Part model, mm, in its own coordinate system. A direction names the side the tool comes from. Round coordinates to 2 decimals unless told otherwise and drop trailing zeros. Loops run counter-clockwise (first coordinate to the right, second up) from the corner with the lowest first, then second, coordinate; pieces in that order, holes last. Notation, with made-up numbers: M 1.5,35 L 57.5,35 A30 ccw 57.5,59 Z; hole C 13.5,4 d3. An arc over 180 degrees is marked long. Answer as CSV lines item,"result". Start each with the question number.
Item 1: Mould opens along X. For faces 1 (the flat face through (0, -30.48, 2)), 2 (the cylindrical face through (-0.34, -33.61, 1.55)), 3 (the flat face through (12, -3.175, 26)) say: pulls with the +X half, pulls with the -X half, needs draft (parallel to the pull), parting line crosses it, or undercut.
Item 2: Band-saw the part on C-C (y = -33). Give the cut face in (x, z) (1 decimal).
Item 3: Band-saw the part on B-B (z = 16.5). Give the cut face in (x, y) (3 decimals).
Item 4: Drop flat-ended pins along their axis: pin 1 Ø5 at (x, y) = (-5.5, -15.5) entering from +Z; pin 2 Ø1 at (y, z) = (-27, 5.5) entering from +X; pin 3 Ø4 at (x, z) = (16.5, 2.5) entering from -Y. Give the stop position or say it passes through.
Item 5: Wall check: line 1 (X direction, y = 1.45, z = 0); line 2 (Y direction, x = -3.5, z = -3). Give the ranges that are in metal, low to high.
Item 6: Which spindle directions (+Z, -Z, +X, -X, +Y, -Y) get a long thin tool onto all of the face, cutting with end or side? Do faces 4 (the flat face through (6, 3.175, 25)), 5 (the flat face through (0, 0, 0)). Say none if no direction does.
Item 7: Band-saw the part on D-D (x = -10). Give the cut face in (y, z) (3 decimals).
Autodesk Inventor part; units mm, degrees
ref_plane "YZ Plane" through (0, 0, 0) normal (1, 0, 0) x (0, 1, 0)
ref_plane "XZ Plane" through (0, 0, 0) normal (0, 1, 0) x (-1, 0, 0)
ref_plane "XY Plane" through (0, 0, 0) normal (0, 0, 1) x (1, 0, 0)
sketch "Sketch1" plane through (0, 0, 0) normal (0, 1, 0) x (-1, 0, 0)
  arc A0 (-31.75, 0) -> (31.75, 0) centre (0, 0) ccw
  line L0 (0, 0) -> (-31.75, 0) construction
  line L1 (0, 0) -> (31.75, 0) construction
  line L2 (31.75, 0) -> (-31.75, 0)
  dimension "d0" = 31.75
  dimension "d1" = 180
revolve "Revolution1" add sketch "Sketch1" angle 180 about axis through (-31.75, 0, 0) along (-1, 0, 0)
sketch "Sketch2" plane through (0, 0, 0) normal (0, 1, 0) x (1, 0, 0)
  line L0 (0, 0) -> (0, 27.94)
  line L1 (0, 27.94) -> (0, 0)
  line L2 (0, 0) -> (0, 25.4)
  circle A0 centre (0, 0) radius 27.94
  circle A1 centre (0, 0) radius 25.4
  dimension "d3" = 27.94
  dimension "d4" = 25.4
extrude "Extrusion1" add sketch "Sketch2" along normal blind 3.175
sketch "Sketch3" plane through (0, 0, 0) normal (0, 1, 0) x (1, 0, 0)
  circle A0 centre (0, 0) radius 27.94
  circle A1 centre (0, 0) radius 31.75
extrude "Extrusion2" cut sketch "Sketch3" against normal blind 3.175
sketch "Sketch4" plane through (0, 0, 0) normal (0, 1, 0) x (1, 0, 0)
  circle A0 centre (0, 0) radius 31.75
  dimension "d9" = 63.5
extrude "Extrusion3" cut sketch "Sketch4" along normal blind 50.8 and the other way blind 30.48 keep common part
sketch "Sketch5" plane through (0, -30.48, 0) normal (0, -1, 0) x (1, 0, 0)
  circle A0 centre (0, 0) radius 1.5875
  dimension "d14" = 3.175
extrude "Extrusion4" add sketch "Sketch5" along normal blind 6.35
properties part number "mid ball bottom"
Answer block:
1,face 1,"needs draft"
1,face 2,"parting line crosses it"
1,face 3,"undercut"
2,outline,"C 0,0 d3.2"
3,outline,"M -26.939,-3.175 A27.126 ccw 26.939,-3.175 L 22.548,-3.175 L 22.548,3.175 L 19.311,3.175 L 19.311,0 L -19.311,0 L -19.311,3.175 L -22.548,3.175 L -22.548,-3.175 Z"
4,pin 1,"stops at z = 28.52"
4,pin 2,"stops at x = 16.62"
4,pin 3,"stops at y = -28.15"
5,line 1,"x = -27.94 to -25.4, 25.4 to 27.94"
5,line 2,"y = -30.48 to 0"
6,face 4,"+Z, -Z, +X, -X, +Y"
6,face 5,"+Y"
7,outline,"M -3.175,-29.966 L -3.175,-26.089 L 3.175,-26.089 L 3.175,-23.349 L 0,-23.349 L 0,23.349 L 3.175,23.349 L 3.175,26.089 L -3.175,26.089 L -3.175,29.966 A30.134 ccw Z"
